```python
from build123d import *

# Parameters (mm, degrees)
CROQUIS2_R                 = 5
CORTAR_EXTRUIR2_DEPTH      = 328.223165581
CORTAR_EXTRUIR2_DEPTH_BACK = 328.223165581
CROQUIS4_R                 = 2.5


with BuildPart() as part:
    # Barrer1: sweep along a path in Croquis1
    with BuildLine(Plane.XY) as barrer1_path:
        Line((0, 0), (0, 180))
        ThreePointArc((0, 180), (5.857864376, 194.142135624), (20, 200))
        Line((20, 200), (230, 200))
        ThreePointArc((230, 200), (244.142135624, 194.142135624), (250, 180))
        Line((250, 180), (250, -100))
    # Croquis2 → Barrer1 (sweep)
    with BuildSketch(Plane(origin=(0, 0, 0), x_dir=(1, 0, 0), z_dir=(0, 1, 0))):
        Circle(CROQUIS2_R)
    sweep(path=barrer1_path.line)

    # Croquis4 → Cortar-Extruir2 (cut, two sides: drawn at the far end of the back side and taken through both)
    with BuildSketch(Plane(origin=(0, 0, 0), x_dir=(0, 0, -1), z_dir=(1, 0, 0)).offset(-CORTAR_EXTRUIR2_DEPTH_BACK)):
        with Locations((0, 52.5)):
            Circle(CROQUIS4_R)
    extrude(amount=CORTAR_EXTRUIR2_DEPTH + CORTAR_EXTRUIR2_DEPTH_BACK, mode=Mode.SUBTRACT)


solid = part.part
```
Geometry check sheet. Reference: the model listing, model coordinates, mm. A direction names the side the tool comes from. Coordinates: 2 decimals unless noted, no trailing zeros. Order: outer loops, then holes, each group sorted by start corner. A loop starts at its lowest first (then second) coordinate and runs counter-clockwise, first axis right, second up. Notation, with made-up numbers: M 13.5,33 L 71.5,33 A17 cw 71.5,54 Z; hole C -35.5,-4.75 d2. An arc over 180 degrees is marked long. One line per question, with ' | ' between items. Start each with the question number.
Item 1: Cross-section at B-B on y = 100. Enter the section's corners in (x, z), then the cut area to 3 significant figures.
Item 2: Cross-section at C-C on x = 173. Enter the section's corners in (y, z).
Item 3: Draft check along X on faces 4 (the cylindrical face through (245.23, 38.04, -1.5)), 5 (the flat face through (250, -100, 0)). Enter one of: pulls with the +X half, pulls with the -X half, needs draft (parallel to the pull), parting line crosses it, or undercut.
Item 4: Cross-section at D-D on y = -48. Enter the section's corners in (x, z), then the cut area to 3 significant figures.
Item 5: Gauge pin test, flat ends, axial feed: pin 1 (3 mm diameter, centred on x = 2, z = 1.5, fed in from -Y); pin 2 (2 mm diameter, centred on x = 160, z = -3.5, fed in from +Y); pin 3 (4.5 mm diameter, centred on y = 52.5, z = 0, fed in from +X); pin 4 (1.5 mm diameter, centred on x = 184.5, z = -2, fed in from +Y). Record the tip position at first contact, or that the pin passes through.
Item 6: Material ranges on L1, parallel to Y at x = 250.25, z = 0; L2, parallel to Z at x = 247.25, y = 52.5; L3, parallel to X at y = 54.5, z = 3.75, recorded low to high. Write a range as [from, to].
Item 7: Set-up check for faces 1 (the flat face through (0, 0, 0)), 2 (the cylindrical face through (126.47, 195.23, -1.5)), 3 (the cylindrical face through (-5, 91, 0)): record each of +Z, -Z, +X, -X, +Y, -Y from which the full face is reachable in a straight line by a thin tool's end or side.
Item 8: Cross-section at A-A on z = 0. Enter the section's corners in (x, y), then the cut area to 3 significant figures.
Findings:
1) outline: C 0,0 d10; C 250,0 d10 | area: 157 mm²
2) outline: C 200,0 d10
3) face 4: undercut | face 5: needs draft
4) outline: C 250,0 d10 | area: 78.5 mm²
5) pin 1: stops at y = 0 | pin 2: stops at y = 204.33 | pin 3: passes through | pin 4: stops at y = 204.84
6) L1: y = [-100, 50], [55, 194.66] | L2: z = [-4.18, -2.5], [2.5, 4.18] | L3: x = [-3.31, 3.31], [246.69, 253.31]
7) face 1: +Z, -Z, -X, -Y | face 2: none | face 3: -Y
8) outline: M -5,0 L 5,0 L 5,50 L -5,50 Z; M -5,55 L 5,55 L 5,180 A15 cw 20,195 L 230,195 A15 cw 245,180 L 245,55 L 255,55 L 255,180 A25 ccw 230,205 L 20,205 A25 ccw -5,180 Z; M 245,-100 L 255,-100 L 255,50 L 245,50 Z | area: 7,230 mm²
